Could you check a few things on this drawing? It's one solid part, dimensions in mm from its lowest x, y, z. A direction names the side the tool comes from. Give positions to 0.01 mm unless a question says otherwise; leave off trailing zeros. Loops run counter-clockwise (first coordinate to the right, second up) from the corner with the lowest first, then second, coordinate; pieces in that order, holes last.
Q1. I'm going to push flat-ended pins straight in: P1, Ø12, axis at y = 245.5, z = 114.5, coming from the -X side; P2, Ø1, axis at x = 117.5, y = 226, coming from the -Z side; P3, Ø4, axis at x = 78, z = 220.5, coming from the -Y side. Where does each tip first touch, or does it pass through?
Q2. I need wall thicknesses on probe 1 along Y at (x, z) = (114.5, 160); probe 2 along X at (y, z) = (94, 133); probe 3 along X at (y, z) = (154.5, 26.5). Which ranges of each line are inside material? Lowest first, please.
Q3. For the marked faces 4, 5 and 6, which set-ups out of +Z, -Z, +X, -X, +Y, -Y let a thin tool reach every point of the face, with its end or its side?
Q4. Thinking about a two-plate mould opening in X: for the marked faces 1, 2 and 3, which applies, pulls with the +X half, pulls with the -X half, needs draft (parallel to the pull), parting line crosses it, or undercut?
Q5. Suppose I cut it at D-D (x = 21). List the corners of the cut face in (y, z) for me, and give its area (3 significant figures).
Q6. Suppose I cut it at C-C (x = 114.5). List the corners of the cut face in (y, z) for me.
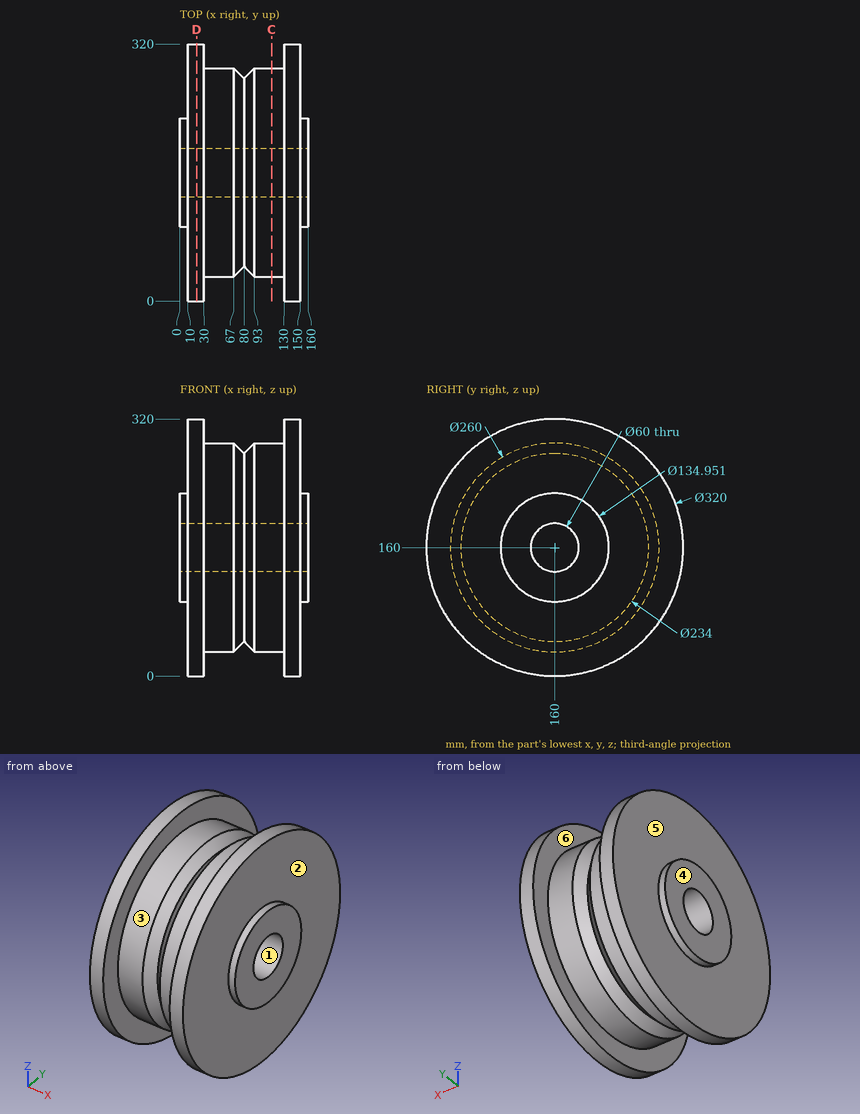
Solutions:
1. P1: stops at x = 10
1. P2: stops at z = 47.71
1. P3: stops at y = 54.94
2. probe 1: y = 30 to 130, 190 to 290
2. probe 2: x = 10 to 150
2. probe 3: x = 10 to 30, 130 to 150
3. face 4: +Z, -Z, -X, +Y, -Y
3. face 5: -X
3. face 6: none
4. face 1: needs draft
4. face 2: pulls with the +X half
4. face 3: undercut
5. outline: circle Ø320 at (160, 160); hole circle Ø60 at (160, 160)
5. area: 77,600 mm2
6. outline: circle Ø260 at (160, 160); hole circle Ø60 at (160, 160)
